```python
from build123d import *

# Parameters (mm, degrees)
BOSS_EXTRUDE1_DEPTH = 3.5
SKETCH2_R           = 0.8
SCREW_HOLES_DEPTH   = 37.028935124
SKETCH3_W           = 4
SKETCH3_H           = 14
BOSS_EXTRUDE2_DEPTH = 8
WIRE_CANAL_DEPTH    = 1.5
CUT_EXTRUDE2_START  = 13
SKETCH5_R           = 0.8
CUT_EXTRUDE2_DEPTH  = 50.74008936
FILLET1_R           = 3.5


with BuildPart() as part:
    # Sketch1 → Boss-Extrude1 (new body)
    with BuildSketch(Plane(origin=(0, 0, 0), x_dir=(1, 0, 0), z_dir=(0, 1, 0))):
        with BuildLine():
            Line((17, -10), (17, -12.105263158))
            Line((17, -12.105263158), (26, -11.631578947))
            Line((26, -11.631578947), (26, 0))
            ThreePointArc((26, 0), (28.126845638, 6.820617489), (33.753470489, 11.223501553))
            Line((33.753470489, 11.223501553), (17, 12.105263158))
            Line((17, 12.105263158), (17, 10))
            Line((17, 10), (17, 7))
            Line((17, 7), (13, 7))
            Line((13, 7), (13, 0))
            Line((13, 0), (13, -7))
            Line((13, -7), (17, -7))
            Line((17, -7), (17, -10))
        make_face()
    extrude(amount=BOSS_EXTRUDE1_DEPTH)

    # Sketch2 → Screw Holes (cut, through all)
    with BuildSketch(Plane(origin=(0, 0, 0), x_dir=(1, 0, 0), z_dir=(0, 1, 0))):
        with Locations(Location((24, 8.5, 0), (0, 0, 270))):
            Circle(SKETCH2_R)
        with Locations(Location((24, 0, 0), (0, 0, 270))):
            Circle(SKETCH2_R)
        with Locations(Location((24, -8.5, 0), (0, 0, 270))):
            Circle(SKETCH2_R)
    extrude(amount=SCREW_HOLES_DEPTH, mode=Mode.SUBTRACT)

    # Sketch3 → Boss-Extrude2 (add)
    with BuildSketch(Plane(origin=(0, 0, 0), x_dir=(1, 0, 0), z_dir=(0, 1, 0))):
        with Locations((15, 0)):
            Rectangle(SKETCH3_W, SKETCH3_H)
    extrude(amount=BOSS_EXTRUDE2_DEPTH)

    # Sketch4 → Wire Canal (cut)
    with BuildSketch(Plane(origin=(0, 0, 0), x_dir=(1, 0, 0), z_dir=(0, 1, 0))):
        Polygon((13, 0), (13, 3), (26.381049961, 3), (26.381049961, -3), (13, -3), align=None)
    extrude(amount=WIRE_CANAL_DEPTH, mode=Mode.SUBTRACT)

    # Sketch5 → Cut-Extrude2 (cut, through all)
    with BuildSketch(Plane.XY.offset(CUT_EXTRUDE2_START)):
        with Locations(Location((15, 6, 0), (0, 0, 180))):
            Circle(SKETCH5_R)
    extrude(amount=-CUT_EXTRUDE2_DEPTH, mode=Mode.SUBTRACT)

    # Fillet1
    # the kernel refuses this fillet: 3.5 mm, written as the material it takes off along each edge
    with BuildSketch(Plane(origin=(8.262093993, 3.5, 12.565152948), x_dir=(0, -1, 0), z_dir=(0.9986178293325098, 0, -0.05255883312276359))) as fillet1_piece_1:
        with BuildLine():
            CenterArc((FILLET1_R, FILLET1_R), FILLET1_R, 180, 90)
            Line((0, FILLET1_R), (0, 0))
            Line((0, 0), (FILLET1_R, 0))
        make_face()
    extrude(amount=26.512456753, mode=Mode.SUBTRACT)
    with BuildSketch(Plane(origin=(42.491376496, 3.5, -10.763611763), x_dir=(-0.05255883312276374, 0, 0.9986178293325098), z_dir=(-0.9986178293325098, 0, -0.05255883312276374))) as fillet1_piece_2:
        with BuildLine():
            CenterArc((FILLET1_R, -FILLET1_R), FILLET1_R, 90, 90)
            Line((0, -FILLET1_R), (0, 0))
            Line((0, 0), (FILLET1_R, 0))
        make_face()
    extrude(amount=34.276658695, mode=Mode.SUBTRACT)


solid = part.part
```
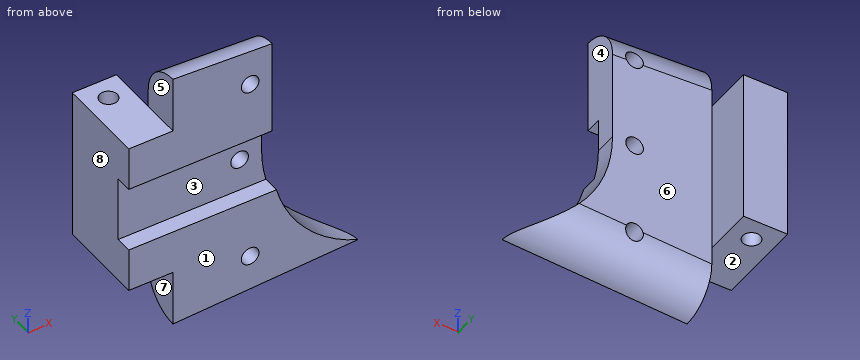
Geometry check sheet. Reference: the model listing, model coordinates, mm. Face numbers are marked on the shaded views. A direction names the side the tool comes from. Coordinates: 2 decimals unless noted, no trailing zeros. Loops run counter-clockwise (first coordinate to the right, second up) from the corner with the lowest first, then second, coordinate; pieces in that order, holes last. Notation, with made-up numbers: (63, 77) - (88, 77) arc R17 ccw to (88, 95) - close; hole circle Ø5 at (75.5, -4). An arc over 180 degrees is marked (long way). One line per item, written item: value. Start each with the question number.
(1) Material ranges on line 1 (X direction, y = 2.3, z = 8.5); line 2 (X direction, y = 6, z = -2.75); line 3 (Z direction, x = 24, y = 2.6), recorded low to high. Write a range as [from, to].
(2) Depth check by flat-ended pin: P1, Ø1.8, axis at x = 15, y = 6, coming from the +Z side; P2, Ø3, axis at x = 19, z = -0.5, coming from the -Y side; P3, Ø3, axis at x = 17.5, y = 6, coming from the -Z side. Enter the tip coordinate at first touch or a pass-through.
(3) Mould release check, pull along Z, two halves, no side actions. Record for the marked faces 1, 2 and 3: released by +Z, released by -Z, zero draft, split by the parting line, or undercut.
(4) Cross-section at A-A on y = 0.75. Enter the section's corners in (x, z).
(5) Cross-section at D-D on z = 2.25. Enter the section's corners in (x, y), plus the area to 3 significant figures.
(6) Cross-section at C-C on x = 15. Enter the section's corners in (y, z), plus the area to 3 significant figures.
(7) Tool access check on the marked faces 4, 5, 6, 7 and 8. Record the directions out of +Z, -Z, +X, -X, +Y, -Y that give a thin tool (end or side, any length) a straight path to the whole face; none if there is none.
(8) Cross-section at B-B on z = 5. Enter the section's corners in (x, y), plus the area to 3 significant figures.
Results below:
1. line 1: x = [17, 23.2], [24.8, 26]
1. line 2: x = [13, 14.2], [15.8, 17]
1. line 3: z = [-10.58, -9.3], [-7.7, -0.8], [0.8, 7.7], [9.3, 10.58]
2. P1: stops at z = 7
2. P2: stops at y = 1.5
2. P3: stops at z = -7
3. face 1: zero draft
3. face 2: released by -Z
3. face 3: undercut
4. outline: (13, -7) - (17, -7) - (17, -12.02) - (33.57, -11.15) arc R12 cw to (26.38, -3) - (13, -3) - close; (13, 3) - (26, 3) - (26, 11.55) - (17, 12.02) - (17, 7) - (13, 7) - close; hole circle Ø1.6 at (24, -8.5); hole circle Ø1.6 at (24, 8.5)
5. outline: (13, 1.5) - (26, 1.5) - (26, 3.5) - (17, 3.5) - (17, 8) - (13, 8) - close; hole circle Ø1.6 at (15, 6)
5. area: 42.0 mm2
6. outline: (0, -7) - (5.2, -7) - (5.2, 7) - (0, 7) - (0, 3) - (1.5, 3) - (1.5, -3) - (0, -3) - close; (6.8, -7) - (8, -7) - (8, 7) - (6.8, 7) - close
6. area: 80.6 mm2
7. face 4: +Z, +X, +Y, -Y
7. face 5: +Z, -X, +Y, -Y
7. face 6: +Z, -Z, +X, +Y
7. face 7: -Z, -X, +Y, -Y
7. face 8: +Z, -Z, -X, +Y, -Y
8. outline: (13, 0) - (26, 0) - (26, 3.5) - (17, 3.5) - (17, 8) - (13, 8) - close; hole circle Ø1.6 at (15, 6)
8. area: 61.5 mm2
